from build123d import *

# Parameters (mm, degrees)
SKETCH1_W           = 53.32
SKETCH1_H           = 79.98
BOSS_EXTRUDE1_DEPTH = 5.08
SKETCH2_W           = 5.08
SKETCH2_H           = 5.08
BOSS_EXTRUDE2_DEPTH = 5.08


with BuildPart() as part:
    # Sketch1 → Boss-Extrude1 (new body)
    with BuildSketch(Plane.XY):
        with Locations((19.705217391, 3.361478261)):
            Rectangle(SKETCH1_W, SKETCH1_H)
    extrude(amount=BOSS_EXTRUDE1_DEPTH)

    # Sketch2 → Boss-Extrude2 (add)
    with BuildSketch(Plane.XY.offset(5.08)):
        with Locations((1.925217391, 45.891478261)):
            Rectangle(SKETCH2_W, SKETCH2_H)
        with Locations((27.325217391, 45.891478261)):
            Rectangle(SKETCH2_W, SKETCH2_H)
        with Locations((37.485217391, 45.891478261)):
            Rectangle(SKETCH2_W, SKETCH2_H)
        with Locations((12.085217391, 45.891478261)):
            Rectangle(SKETCH2_W, SKETCH2_H)
        with Locations((12.085217391, -39.168521739)):
            Rectangle(SKETCH2_W, SKETCH2_H)
        with Locations((1.925217391, -39.168521739)):
            Rectangle(SKETCH2_W, SKETCH2_H)
        with Locations((37.485217391, -39.168521739)):
            Rectangle(SKETCH2_W, SKETCH2_H)
        with Locations((27.325217391, -39.168521739)):
            Rectangle(SKETCH2_W, SKETCH2_H)
    extrude(amount=-BOSS_EXTRUDE2_DEPTH)


solid = part.part
Part model, mm, in its own coordinate system. A direction names the side the tool comes from. Give positions to 0.01 mm unless a question says otherwise; leave off trailing zeros. Order: outer loops, then holes, each group sorted by start corner. A loop starts at its lowest first (then second) coordinate and runs counter-clockwise, first axis right, second up. Notation, with made-up numbers: (36, -5) - (57, -5) arc R31 ccw to (57, 26) - close; hole circle Ø3 at (0, -36.5). An arc over 180 degrees is marked (long way). One line per question, with ' | ' between items.
1. Drop flat-ended pins along their axis: P1, Ø1.5, axis at y = 44.5, z = 1.5, coming from the +X side; P2, Ø1.5, axis at y = -40, z = 3.5, coming from the -X side; P3, Ø2.5, axis at x = 20, z = 1.5, coming from the +Y side; P4, Ø8, axis at x = 36, y = 3.5, coming from the -Z side. Give the stop position or say it passes through.
Filled in:
P1: x = 40.03 | P2: x = -0.61 | P3: y = 43.35 | P4: z = 0
2. Pull direction X, two halves, no side cores. Call faces 1 (the face through (27, -41.709, 3)), 2 (the face through (40.025, -39, 3)), 3 (the face through (7, 43.351, 3)): +X half, -X half, draft (parallel to the pull), parting line (faces both ways), or undercut.
Filled in:
face 1: draft | face 2: +X half | face 3: undercut
3. Which spindle directions (+Z, -Z, +X, -X, +Y, -Y) get a long thin tool onto all of the face, cutting with end or side? Do faces 4 (the face through (43, 43.351, 3)), 5 (the face through (43, -36.629, 3)), 6 (the face through (32, -36.629, 3)), 7 (the face through (46.365, 3, 3)), 8 (the face through (34.945, 46, 3)). Say none if no direction does.
Filled in:
face 4: +Z, -Z, +X, +Y | face 5: +Z, -Z, +X, -Y | face 6: +Z, -Z, -Y | face 7: +Z, -Z, +X, +Y, -Y | face 8: +Z, -Z, +Y
4. Band-saw the part on A-A on x = 33. List the corners of the cut face in (y, z), then the cut area to 3 significant figures.
Filled in:
outline: (-36.63, 0) - (43.35, 0) - (43.35, 5.08) - (-36.63, 5.08) - close | area: 406 mm²
5. Drill centre lines: probe 1 along X at (y, z) = (44, 0.95); probe 2 along Y at (x, z) = (-1, 0.45). Where is each one in solid material? Low to high.
Filled in:
probe 1: -0.61 to 4.47, 9.55 to 14.63, 24.79 to 29.87, 34.95 to 40.03 | probe 2: -36.63 to 43.35
